For this review, take the finished solid that the model builds, in its own axes (mm). Give positions to 0.01 mm unless a question says otherwise; leave off trailing zeros. Write each loop counter-clockwise with the first axis right and the second up, starting at its lowest first coordinate (ties: lowest second). Pieces come first, ordered by that corner, then holes. Notation, with made-up numbers: (77, -24) -> (116, -24) arc R18 ccw to (116, -7) -> close; hole circle Ø6 at (5.5, 2). An arc over 180 degrees is marked (long way). Write item = value, one per line.
Autodesk Inventor part; units mm, degrees
ref_plane "YZ Plane" through (0, 0, 0) normal (1, 0, 0) x (0, 1, 0)
ref_plane "XZ Plane" through (0, 0, 0) normal (0, 1, 0) x (-1, 0, 0)
ref_plane "XY Plane" through (0, 0, 0) normal (0, 0, 1) x (1, 0, 0)
sketch "Sketch1" plane through (0, 0, 0) normal (0, 0, 1) x (1, 0, 0)
  line L0 (-75, -42.5) -> (75, -42.5)
  line L1 (75, -42.5) -> (75, 42.5)
  line L2 (75, 42.5) -> (-75, 42.5)
  line L3 (-75, 42.5) -> (-75, -42.5)
  line L4 (-75, -42.5) -> (75, 42.5) construction
  line L5 (75, -42.5) -> (-75, 42.5) construction
  circle A0 centre (55, -22.5) radius 8.5
  circle A1 centre (55, 22.5) radius 8.5
  line L6 (0, 0) -> (75, 0) construction
  circle A2 centre (55, 0) radius 8.5
  dimension "d0" = 150
  dimension "d1" = 85
  dimension "d23" = 17
  dimension "d25" = 20
  dimension "d26" = 20
extrude "Plate1" add sketch "Sketch1" along normal blind 6 contours L3 L2 L1 L0 | A0 | A1
sketch "Sketch5" plane through (0, 0, 6) normal (0, 0, 1) x (1, 0, 0)
  line L0 (75, -42.5) -> (-75, -42.5)
  line L1 (-75, -42.5) -> (-75, 42.5)
  line L2 (-75, 42.5) -> (75, 42.5)
  circle A0 centre (-32.5, 0) radius 42.5
  circle A1 centre (-32.5, 0) radius 5
  point P0 (0, 0)
  point P1 (50, -55)
  point P2 (-50, -55)
  point P3 (-70, -35)
  point P4 (-70, 35)
  point P5 (-50, 55)
  point P6 (50, 55)
  dimension "d27" = 10
extrude "Extrusion2" [suppressed]
fillet "Corner Round2" radius 5 4 edges at (-75, 42.5, 3) (-75, -42.5, 3) (75, -42.5, 3) (75, 42.5, 3)
equation "\"d26\" = d25"
equation "\"d2\" = Thickness"
equation "\"BendReliefWidth\" = Thickness"
equation "\"BendReliefDepth\" = 0.5 * Thickness"
equation "\"CornerReliefSize\" = 4 * Thickness"
equation "\"MinimumRemnant\" = 2 * Thickness"
equation "\"TransitionRadius\" = BendRadius"
equation "\"JacobiRadiusSize\" = BendRadius"
equation "\"GapSize\" = Thickness"
properties part number "SLM 1695 leg floor plate" material "Stainless Steel"
(1) Take a section at A-A (z = 4.55). Write out the cut boundary in (x, y), plus the area to 3 significant figures.
Answers below:
outline = (-75, -37.5) arc R5 ccw to (-70, -42.5) -> (70, -42.5) arc R5 ccw to (75, -37.5) -> (75, 37.5) arc R5 ccw to (70, 42.5) -> (-70, 42.5) arc R5 ccw to (-75, 37.5) -> close; hole circle Ø17 at (55, 0)
area = 12,500 mm^2
(2) Take a section at B-B (x = 55). Write out the cut boundary in (y, z).
Answers below:
outline = (-42.5, 0) -> (-8.5, 0) -> (-8.5, 6) -> (-42.5, 6) -> close; (8.5, 0) -> (42.5, 0) -> (42.5, 6) -> (8.5, 6) -> close
(3) Take a section at C-C (y = 0). Write out the cut boundary in (x, z).
Answers below:
outline = (-75, 0) -> (46.5, 0) -> (46.5, 6) -> (-75, 6) -> close; (63.5, 0) -> (75, 0) -> (75, 6) -> (63.5, 6) -> close
(4) The part is to be moulded in two halves that separate along Y. For faces 1 (the face through (46.51, -0.37, 2.96)), 2 (the face through (73.57, 41, 3.04)), 3 (the face through (-1, 1, 6)), say which applies: released by +Y, released by -Y, zero draft, split by the parting line, or undercut.
Answers below:
face_1 = undercut
face_2 = released by +Y
face_3 = zero draft
(5) To check wall thickness, follow probe 1 along Y at (x, z) = (55, 2.5); probe 2 along Y at (x, z) = (59.5, 0.75); probe 3 along X at (y, z) = (-2.5, 4.7). State the ranges of each line that lie inside material, in increasing order.
Answers below:
probe_1 = -42.5 to -8.5, 8.5 to 42.5
probe_2 = -42.5 to -7.21, 7.21 to 42.5
probe_3 = -75 to 46.88, 63.12 to 75
